For this review, take the finished solid that the model builds, in its own axes (mm). A direction names the side the tool comes from. Coordinates: 2 decimals unless noted, no trailing zeros. Loops run counter-clockwise (first coordinate to the right, second up) from the corner with the lowest first, then second, coordinate; pieces in that order, holes last. Notation, with made-up numbers: (65.5, 22) - (83.5, 22) arc R24 cw to (83.5, 35) - close; hole circle Ø7 at (2, -7.75). An arc over 180 degrees is marked (long way). One line per item, written item: value. Start each with the question number.
1. Take a section at A-A, the plane z = 12. State the section outline as (x, y) points.
2. Take a section at B-B, the plane x = -27. State the section outline as (y, z) points.
3. The part is to be moulded in two halves that separate along Y. For faces 1 (the face through (-2.003, 0.631, 31.443)), 2 (the face through (1, -4.953, 11)), 3 (the face through (-26.035, 0, 30)), say which applies: released by +Y, released by -Y, zero draft, split by the parting line, or undercut.
4. For faces 4 (the face through (46.393, 0, -2)), 5 (the face through (17.12, 0, -2)), 6 (the face through (36, 0, 25.4)), 7 (the face through (12.1, 0.09, 31.44)), list the 3-axis set-ups (+Z, -Z, +X, -X, +Y, -Y) from which the entire face can be reached by the end or side of a thin tool; tool diameter is ignored.
5. Insertion check: pin 1 (0.9 mm diameter, centred on y = 1.5, z = -2.5, fed in from +X); pin 2 (0.9 mm diameter, centred on y = 1.5, z = -3, fed in from -X); pin 3 (12 mm diameter, centred on x = -32, z = 9.5, fed in from -Y); pin 4 (3 mm diameter, centred on x = -4.953, z = 28.956, fed in from +Y). Each pin has a flat end and moves straight along its axis. Give the tip position at first contact, or say it passes through.
6. To check wall thickness, follow line 1 (Y direction, x = 10, z = 30); line 2 (X direction, y = 0, z = 30.75) (3 decimals); line 3 (X direction, y = 2.5, z = -0.5). State the ranges of each line that lie inside material, in increasing order. Write a range as from..to.
```python
from build123d import *

# Parameters (mm, degrees)
BOSS_EXTRUDE1_DEPTH                 = 4.953
SKETCH4_W                           = 52.07
SKETCH4_H                           = 9.906
BOSS_EXTRUDE3_DEPTH                 = 6.0325
SKETCH5_R                           = 1.6129
CUT_EXTRUDE1_DEPTH                  = 12.065
M5X0_8_TAPPED_HOLE1_D               = 4.2
M5X0_8_TAPPED_HOLE1_DEPTH           = 7.62
M5X0_8_TAPPED_HOLE1_TIP             = 1.2618073
M5X0_8_TAPPED_HOLE1_ON_FACE_2_D     = 4.2
M5X0_8_TAPPED_HOLE1_ON_FACE_2_DEPTH = 7.62
M5X0_8_TAPPED_HOLE1_ON_FACE_2_TIP   = 1.2618073


with BuildPart() as part:
    # Sketch1 → Boss-Extrude1 (new, symmetric)
    with BuildSketch(Plane(origin=(0, 0, 0), x_dir=(1, 0, 0), z_dir=(0, 1, 0))):
        Polygon((17.1196, 3.81), (46.3931, 3.81), (46.3931, 0.8509), (53.2511, 0.8509), (53.2511, -7.4041), (46.3931, -7.4041), (46.3931, -25.4), (26.035, -25.4), (-26.035, -25.4), (-46.3931, -25.4), (-46.3931, -7.4041), (-53.2511, -7.4041), (-53.2511, 0.8509), (-46.3931, 0.8509), (-46.3931, 3.81), (-17.1196, 3.81), (-17.1196, 0), (17.1196, 0), align=None)
    extrude(amount=BOSS_EXTRUDE1_DEPTH, both=True)

    # Sketch4 → Boss-Extrude3 (add, symmetric)
    with BuildSketch(Plane(origin=(0, 0, 0), x_dir=(1, 0, 0), z_dir=(0, 1, 0))):
        with Locations((0, -30.353)):
            Rectangle(SKETCH4_W, SKETCH4_H)
    extrude(amount=BOSS_EXTRUDE3_DEPTH, both=True)

    # Sketch5 → Cut-Extrude1 (cut)
    with BuildSketch(Plane(origin=(0, 6.0325, 0), x_dir=(1, 0, 0), z_dir=(0, 1, 0))):
        with Locations(Location((-4.953, -28.956, 0), (0, 0, 270))):
            Circle(SKETCH5_R)
        with Locations(Location((4.953, -28.956, 0), (0, 0, 270))):
            Circle(SKETCH5_R)
    extrude(amount=-CUT_EXTRUDE1_DEPTH, mode=Mode.SUBTRACT)

    # M5x0.8 Tapped Hole1
    with Locations(Plane.XY.offset(35.306)):
        with Locations((0, 0), (-10, 0), (10, 0)):
            Hole(M5X0_8_TAPPED_HOLE1_D / 2, depth=M5X0_8_TAPPED_HOLE1_DEPTH)
            with Locations((0, 0, -(M5X0_8_TAPPED_HOLE1_DEPTH + M5X0_8_TAPPED_HOLE1_TIP / 2))):  # 118° drill point
                Cone(0, M5X0_8_TAPPED_HOLE1_D / 2, M5X0_8_TAPPED_HOLE1_TIP, mode=Mode.SUBTRACT)

    # M5x0.8 Tapped Hole1 on face 2
    with Locations(Plane(origin=(-5, 0, 0), x_dir=(-1, 0, 0), z_dir=(0, 0, -1))):
        with Locations((0, 0), (-10, 0)):
            Hole(M5X0_8_TAPPED_HOLE1_ON_FACE_2_D / 2, depth=M5X0_8_TAPPED_HOLE1_ON_FACE_2_DEPTH)
            with Locations((0, 0, -(M5X0_8_TAPPED_HOLE1_ON_FACE_2_DEPTH + M5X0_8_TAPPED_HOLE1_ON_FACE_2_TIP / 2))):  # 118° drill point
                Cone(0, M5X0_8_TAPPED_HOLE1_ON_FACE_2_D / 2, M5X0_8_TAPPED_HOLE1_ON_FACE_2_TIP, mode=Mode.SUBTRACT)


solid = part.part
```
Solutions:
1. outline: (-46.39, -4.95) - (46.39, -4.95) - (46.39, 4.95) - (-46.39, 4.95) - close
2. outline: (-4.95, -3.81) - (4.95, -3.81) - (4.95, 25.4) - (-4.95, 25.4) - close
3. face 1: undercut
3. face 2: released by -Y
3. face 3: zero draft
4. face 4: -Z, +X, +Y, -Y
4. face 5: -Z, +Y, -Y
4. face 6: +Z, +X, +Y, -Y
4. face 7: +Z
5. pin 1: x = 46.39
5. pin 2: x = -46.39
5. pin 3: y = -4.95
5. pin 4: through
6. line 1: -6.03..-2.1, 2.1..6.03
6. line 2: -26.035..-12.1, -7.9..-2.1, 2.1..7.9, 12.1..26.035
6. line 3: -53.25..-17.12, 17.12..53.25
